Autodesk Inventor part; units mm, degrees
ref_plane "YZ Plane" through (0, 0, 0) normal (1, 0, 0) x (0, 1, 0)
ref_plane "XZ Plane" through (0, 0, 0) normal (0, 1, 0) x (-1, 0, 0)
ref_plane "XY Plane" through (0, 0, 0) normal (0, 0, 1) x (1, 0, 0)
sketch "Esquisse1" plane through (0, 0, 0) normal (1, 0, 0) x (0, 1, 0)
  line L0 (0, 0) -> (25, 0)
  line L1 (25, 0) -> (25, -30)
  line L2 (25, -30) -> (0, -30)
  line L3 (0, -30) -> (0, 0)
  dimension "d0" = 25
  dimension "d1" = 30
extrude "Extrusion1" add sketch "Esquisse1" along normal blind 265
sketch "Esquisse2" plane through (0, 25, 0) normal (0, 1, 0) x (1, 0, 0)
  circle A0 centre (15, 15) radius 1.5
  line L0 (0, 30) -> (0, 0)
  circle A1 centre (255, 15) radius 1.5
  dimension "d4" = 3
  dimension "d5" = 15
  dimension "d6" = 240
  dimension "d9" = 3
extrude "Extrusion2" cut sketch "Esquisse2" against normal through all
sketch "Esquisse3" plane through (0, 0, 0) normal (0, 0, 1) x (1, 0, 0)
  line L0 (0, 25) -> (265, 25)
  line L1 (0, 25) -> (40, 25)
  line L2 (40, 25) -> (40, 12.5)
  line L3 (40, 12.5) -> (0, 12.5)
  line L4 (0, 12.5) -> (0, 25)
  line L5 (265, 25) -> (225, 25)
  line L6 (225, 25) -> (225, 12.5)
  line L7 (225, 12.5) -> (265, 12.5)
  line L8 (265, 12.5) -> (265, 25)
  point P0 (0, 0)
  dimension "d10" = 12.5
  dimension "d11" = 40
  dimension "d12" = 40
extrude "Extrusion3" cut sketch "Esquisse3" against normal through all
properties part number "Bras_arrierre"
Part model, mm, in its own coordinate system. A direction names the side the tool comes from. Give positions to 0.01 mm unless a question says otherwise; leave off trailing zeros. Write each loop counter-clockwise with the first axis right and the second up, starting at its lowest first coordinate (ties: lowest second). Pieces come first, ordered by that corner, then holes. Notation, with made-up numbers: M 63,54 L 106,54 A36 cw 106,91 Z; hole C 49,15 d4. An arc over 180 degrees is marked long. Use CSV: the item, a comma, the result in double quotes.
Item 1: Drill centre lines: probe 1 along X at (y, z) = (4, -15); probe 2 along Z at (x, y) = (15, 3); probe 3 along X at (y, z) = (11.5, -14.5). Where is each one in solid material? Low to high.
Taken from the geometry:
probe 1,"x = 0 to 13.5, 16.5 to 253.5, 256.5 to 265"
probe 2,"z = -30 to -16.5, -13.5 to 0"
probe 3,"x = 0 to 13.59, 16.41 to 253.59, 256.41 to 265"
Item 2: Pin check, flat tips, straight feed: P1, Ø2.5, axis at x = 15, z = -15, coming from the -Y side; P2, Ø15, axis at x = 249.5, z = -15, coming from the +Y side; P3, Ø3, axis at y = 16.5, z = -11, coming from the -X side; P4, Ø1, axis at y = 22, z = -10.5, coming from the +X side. Stop position of each tip, or through.
Taken from the geometry:
P1,"passes through"
P2,"stops at y = 12.5"
P3,"stops at x = 40"
P4,"stops at x = 225"
Item 3: Slice it at A-A on z = -22.25. Write the cut outline in (x, y), plus the area to 4 significant figures.
Taken from the geometry:
outline,"M 0,0 L 265,0 L 265,12.5 L 225,12.5 L 225,25 L 40,25 L 40,12.5 L 0,12.5 Z"
area,"5,625 mm²"
Item 4: Which spindle directions (+Z, -Z, +X, -X, +Y, -Y) get a long thin tool onto all of the face, cutting with end or side? Do faces 1 (the face through (0, 6, -15)), 2 (the face through (20, 12.5, -15)), 3 (the face through (225, 19, -15)). Say none if no direction does.
Taken from the geometry:
face 1,"+Z, -Z, -X, +Y, -Y"
face 2,"+Z, -Z, -X, +Y"
face 3,"+Z, -Z, +X, +Y"
Item 5: Slice it at B-B on y = 19.25. Write the cut outline in (x, z), plus the area to 3 significant figures.
Taken from the geometry:
outline,"M 40,-30 L 225,-30 L 225,0 L 40,0 Z"
area,"5,550 mm²"
Item 6: Pull direction X, two halves, no side cores. Call faces 4 (the face through (265, 6, -15)), 5 (the face through (245, 12.5, -15)), 6 (the face through (40, 19, -15)): +X half, -X half, draft (parallel to the pull), parting line (faces both ways), or undercut.
Taken from the geometry:
face 4,"+X half"
face 5,"draft"
face 6,"-X half"
